Design review of the part built by this model. Coordinates are the model's own, in mm. A direction names the side the tool comes from. Give positions to 0.01 mm unless a question says otherwise; leave off trailing zeros. Write each loop counter-clockwise with the first axis right and the second up, starting at its lowest first coordinate (ties: lowest second). Pieces come first, ordered by that corner, then holes. Notation, with made-up numbers: (-11.5, 65) -> (33.5, 65) arc R21 ccw to (33.5, 91) -> close; hole circle Ø2 at (-32, 87.25). An arc over 180 degrees is marked (long way). Return JSON: item names as keys, results as strings. Group by question number.
from build123d import *

# Parameters (mm, degrees)
F1_DEPTH  = 1016
F3_DEPTH  = 609.6
F5_DEPTH  = 609.6
F6_W      = 152.4
F6_H      = 177.8
F7_DEPTH  = 25.4
F8_W      = 406.4
F8_H      = 203.2
F9_DEPTH  = 25.4
F10_W     = 254
F10_H     = 203.2
F10_H_2   = 50.8
F10_W_2   = 152.4
F10_H_3   = 177.8
F11_DEPTH = 25.4
F12_W     = 76.2
F12_H     = 177.8
F13_DEPTH = 25.4


with BuildPart() as f1:
    # F0 (on Front) → F1 (new body)
    with BuildSketch(Plane.XZ):
        Polygon((-304.8, 0), (0, 0), (304.8, 0), (304.8, 279.4), (0, 381), (-304.8, 279.4), align=None)
    extrude(amount=F1_DEPTH)

    # F2 (on face) → F3 (join)
    with BuildSketch(Plane(origin=(0, 0, 0), x_dir=(-1, 0, 0), z_dir=(0, 1, 0))):
        Polygon((-304.8, 381), (-304.8, 0), (304.8, 0), (304.8, 381), (0, 482.6), align=None)
    extrude(amount=F3_DEPTH)

    # F4 (on face) → F5 (join)
    with BuildSketch(Plane(origin=(-304.8, 0, 0), x_dir=(0, -1, 0), z_dir=(-1, 0, 0))):
        Polygon((-609.6, 203.2), (-609.6, 0), (-304.8, 0), (-304.8, 304.8), align=None)
        Polygon((-304.8, 304.8), (-304.8, 0), (0, 0), (0, 203.2), align=None)
    extrude(amount=F5_DEPTH)

    # F6 (on face) → F7 (cut)
    with BuildSketch(Plane.XZ):
        with Locations((-609.6, 88.9)):
            Rectangle(F6_W, F6_H)
    extrude(amount=-F7_DEPTH, mode=Mode.SUBTRACT)

    # F8 (on face) → F9 (cut)
    with BuildSketch(Plane.XZ.offset(1016)):
        with Locations((0, 101.6)):
            Rectangle(F8_W, F8_H)
    extrude(amount=-F9_DEPTH, mode=Mode.SUBTRACT)

    # F10 (on face) → F11 (cut)
    with BuildSketch(Plane(origin=(0, 609.6, 0), x_dir=(-1, 0, 0), z_dir=(0, 1, 0))):
        with Locations((-152.4, 101.6)):
            Rectangle(F10_W, F10_H)
        with Locations((-152.4, 228.6)):
            Rectangle(F10_W, F10_H_2)
        with Locations((609.6, 88.9)):
            Rectangle(F10_W_2, F10_H_3)
    extrude(amount=-F11_DEPTH, mode=Mode.SUBTRACT)

    # F12 (on face) → F13 (cut)
    with BuildSketch(Plane(origin=(-304.8, 0, 0), x_dir=(0, -1, 0), z_dir=(-1, 0, 0))):
        with Locations((825.5, 88.9)):
            Rectangle(F12_W, F12_H)
    extrude(amount=-F13_DEPTH, mode=Mode.SUBTRACT)


solid = f1.part
Q1. Mouldability with a two-part tool opening along Y and no side actions: class faces 1 (the face through (150.3, 300.5, 432.5)), 2 (the face through (-605.3, 455.1, 254.7)), 3 (the face through (4, 0, 382)), 4 (the face through (-279.4, -825, 90)) as +Y half, -Y half, draft (parallel to the pull), parting line (faces both ways), or undercut.
Q2. Take a section at A-A, the plane z = 101. Give the boundary of the cut face in (x, y).
Q3. Take a section at D-D, the plane y = -576. Give the boundary of the cut face in (x, z), plus the area to 3 significant figures.
Q4. Take a section at B-B, the plane y = 255. Give the boundary of the cut face in (x, z).
Q5. Tool access review of faces 5 (the face through (-611, 25.4, 90)), 6 (the face through (154, 584.2, 129)), 7 (the face through (-605.3, 150.3, 253.3)): name each direction out of +Z, -Z, +X, -X, +Y, -Y from which nothing blocks a thin tool from reaching the whole face with its end or side.
Q6. Take a section at C-C, the plane x = 111. Give the boundary of the cut face in (y, z).
Q7. For L1, parallel to X at y = -654.5, z = 144; L2, parallel to X at y = -853, z = 54; L3, parallel to Y at x = -766.5, z = 61, list the stretches that pass through material, from the lowest coordinate up. Write a range as from..to.
Q8. Insertion check: pin 1 (7.5 mm diameter, centred on x = -587.5, y = 8, fed in from -Z); pin 2 (5 mm diameter, centred on x = 42, z = 59.5, fed in from -Y). Each pin has a flat end and moves straight along its axis. Give the tip position at first contact, or say it passes through.
Final values:
{
 "1": {"face 1": "draft", "face 2": "+Y half", "face 3": "-Y half", "face 4": "undercut"},
 "2": {"outline": "(-914.4, 0) -> (-685.8, 0) -> (-685.8, 25.4) -> (-533.4, 25.4) -> (-533.4, 0) -> (-304.8, 0) -> (-304.8, -787.4) -> (-279.4, -787.4) -> (-279.4, -863.6) -> (-304.8, -863.6) -> (-304.8, -1016) -> (-203.2, -1016) -> (-203.2, -990.6) -> (203.2, -990.6) -> (203.2, -1016) -> (304.8, -1016) -> (304.8, 609.6) -> (279.4, 609.6) -> (279.4, 584.2) -> (25.4, 584.2) -> (25.4, 609.6) -> (-533.4, 609.6) -> (-533.4, 584.2) -> (-685.8, 584.2) -> (-685.8, 609.6) -> (-914.4, 609.6) -> close"},
 "3": {"outline": "(-304.8, 0) -> (304.8, 0) -> (304.8, 279.4) -> (0, 381) -> (-304.8, 279.4) -> close", "area": "201,000 mm²"},
 "4": {"outline": "(-914.4, 0) -> (304.8, 0) -> (304.8, 381) -> (0, 482.6) -> (-304.8, 381) -> (-304.8, 288.2) -> (-914.4, 288.2) -> close"},
 "5": {"face 5": "-Z, -Y", "face 6": "-Z, +Y", "face 7": "+Z, -X, -Y"},
 "6": {"outline": "(-1016, 203.2) -> (-990.6, 203.2) -> (-990.6, 0) -> (584.2, 0) -> (584.2, 254) -> (609.6, 254) -> (609.6, 445.6) -> (0, 445.6) -> (0, 344) -> (-1016, 344) -> close"},
 "7": {"L1": "x = -304.8..304.8", "L2": "x = -279.4..304.8", "L3": "y = 0..609.6"},
 "8": {"pin 1": "stops at z = 177.8", "pin 2": "stops at y = -990.6"}
}
